Answer from the drawing. Dimensions are ordinates in mm from the lowest x, y and z of the part. A direction names the side the tool comes from. Give positions to 0.01 mm unless a question says otherwise; leave off trailing zeros. Write each loop counter-clockwise with the first axis right and the second up, starting at its lowest first coordinate (ties: lowest second). Pieces come first, ordered by that corner, then holes. Notation, with made-up numbers: (9, 40) - (44, 40) arc R21 cw to (44, 65) - close; hole circle Ø7 at (73.5, -5.75). An arc over 180 degrees is marked (long way). Write item = value, one per line.
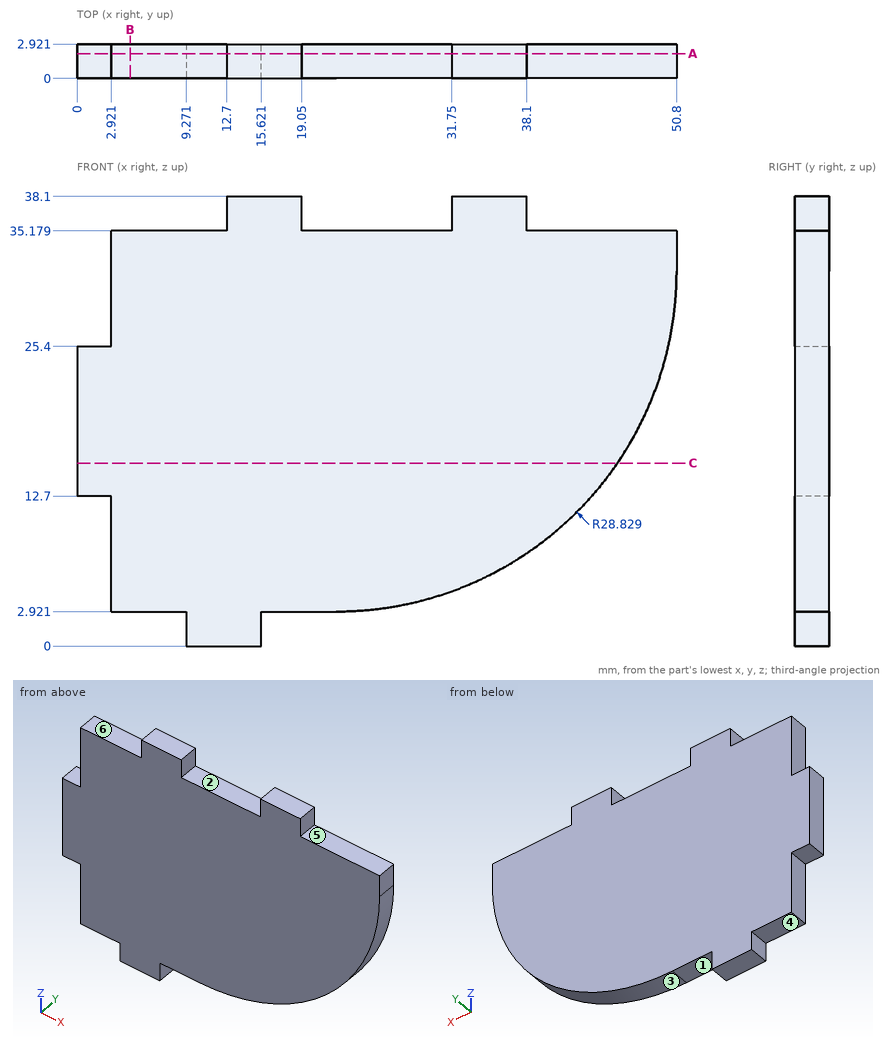
1. For a pull along X with two mould halves and no side action, classify the marked faces 1, 2 and 3 as pulls with the +X half, pulls with the -X half, needs draft (parallel to the pull), parting line crosses it, or undercut.
Solution:
face_1 = needs draft
face_2 = undercut
face_3 = pulls with the +X half
2. Given pin 1 (0.9 mm diameter, centred on y = 1.5, z = 2, fed in from -X); pin 2 (1.5 mm diameter, centred on x = 7.5, y = 1.5, fed in from -Z); pin 3 (0.9 mm diameter, centred on y = 1, z = 28, fed in from -X); pin 4 (3 mm diameter, centred on x = 25.5, z = 11.5, fed in from -Y), each flat-ended and moving along its own axis, determine where each tip first touches the part or whether it passes through.
Solution:
pin_1 = 9.27
pin_2 = 2.92
pin_3 = 2.92
pin_4 = 0
3. Find section A-A, the plane y = 2.1. Give the vertices of the cut face in (x, z), then the cut area to 3 significant figures.
Solution:
outline = (0, 12.7) - (2.92, 12.7) - (2.92, 2.92) - (9.27, 2.92) - (9.27, 0) - (15.62, 0) - (15.62, 2.92) - (21.97, 2.92) arc R28.83 ccw to (50.8, 31.75) - (50.8, 35.18) - (38.1, 35.18) - (38.1, 38.1) - (31.75, 38.1) - (31.75, 35.18) - (19.05, 35.18) - (19.05, 38.1) - (12.7, 38.1) - (12.7, 35.18) - (2.92, 35.18) - (2.92, 25.4) - (0, 25.4) - close
area = 1,460 mm^2
4. Find section C-C, the plane z = 15.5. Give the vertices of the cut face in (x, y), then the cut area to 3 significant figures.
Solution:
outline = (0, 0) - (45.78, 0) - (45.78, 2.92) - (0, 2.92) - close
area = 134 mm^2
5. Find section B-B, the plane x = 4.5. Give the vertices of the cut face in (y, z).
Solution:
outline = (0, 2.92) - (2.92, 2.92) - (2.92, 35.18) - (0, 35.18) - close
6. Straight lines are drawn through the part: line 1 (X direction, y = 2.8, z = 36.5); line 2 (Z direction, x = 9, y = 0.6); line 3 (Z direction, x = 12.5, y = 2.85). For each, find the intervals that lie inside material, in ascending order.
Solution:
line_1 = 12.7 to 19.05, 31.75 to 38.1
line_2 = 2.92 to 35.18
line_3 = 0 to 35.18
7. A tool of negligible diameter and unlimited length cuts with its end or side. For the marked faces 4, 5 and 6, from which of +Z, -Z, +X, -X, +Y, -Y can it reach the whole face along a straight path? Write none if from no direction.
Solution:
face_4 = -Z, -X, +Y, -Y
face_5 = +Z, +X, +Y, -Y
face_6 = +Z, -X, +Y, -Y
